```python
from build123d import *

# Parameters (mm, degrees)
BOSS_EXTRU_1_DEPTH      = 4
ENL_V_MAT_EXTRU_1_REACH = 44.274


with BuildPart() as part:
    # Esquisse1 → Boss.-Extru.1 (new body)
    with BuildSketch(Plane.XY):
        with BuildLine():
            Line((0, 0), (7, 0))
            Line((7, 0), (7, 4))
            Line((7, 4), (8.5, 4))
            add(Edge.make_bspline(
                [(8.5, 4), (8.5, 18.018365096), (18.5, 19.781634904), (18.5, 33.8)],
                knots=[0, 0, 0, 0, 1, 1, 1, 1], degree=3))
            Line((18.5, 33.8), (17, 33.8))
            Line((17, 33.8), (17, 37.8))
            Line((17, 37.8), (10, 37.8))
            Line((10, 37.8), (10, 33.8))
            Line((10, 33.8), (8.5, 33.8))
            add(Edge.make_bspline(
                [(-1.5, 4), (-1.5, 18.018365096), (8.5, 19.781634904), (8.5, 33.8)],
                knots=[0, 0, 0, 0, 1, 1, 1, 1], degree=3))
            Line((-1.5, 4), (0, 4))
            Line((0, 4), (0, 0))
        make_face()
    extrude(amount=BOSS_EXTRU_1_DEPTH)

    # Esquisse2 → Enlèv. mat.-Extru.1 (cut, up to next)
    with BuildSketch(Plane.XY.offset(4), mode=Mode.PRIVATE) as enl_v_mat_extru_1_sk1:
        with BuildLine():
            Line((11.098076211, 32.3), (15.901923789, 32.3))
            add(Edge.make_bspline(
                [(5.901923789, 5.5), (5.901923789, 16.568461709), (15.901923789, 21.231538291), (15.901923789, 32.3)],
                knots=[0, 0, 0, 0, 1, 1, 1, 1], degree=3))
            Line((5.901923789, 5.5), (1.098076211, 5.5))
            add(Edge.make_bspline(
                [(1.098076211, 5.5), (1.098076211, 16.568461709), (11.098076211, 21.231538291), (11.098076211, 32.3)],
                knots=[0, 0, 0, 0, 1, 1, 1, 1], degree=3))
        make_face()
    enl_v_mat_extru_1_tool1 = extrude(enl_v_mat_extru_1_sk1.sketch, amount=-ENL_V_MAT_EXTRU_1_REACH, mode=Mode.PRIVATE) & part.part
    add(enl_v_mat_extru_1_tool1.solids().sort_by_distance((8.5, 18.9, 4))[0], mode=Mode.SUBTRACT)


solid = part.part
```
Verification items for the finished model (mm, model axes). A direction names the side the tool comes from. Round coordinates to 2 decimals unless told otherwise and drop trailing zeros. Loops run counter-clockwise (first coordinate to the right, second up) from the corner with the lowest first, then second, coordinate; pieces in that order, holes last. Notation, with made-up numbers: (0.5, -5.75) -> (19.5, -5.75) arc R11 ccw to (19.5, 0.25) -> close; hole circle Ø11 at (15, 76). An arc over 180 degrees is marked (long way). Answer as a JSON object with one key per item and string values.
Q1. Draft check along X on faces 1 (the flat face through (13, 32.3, 2)), 2 (the flat face through (7, 2, 2)), 3 (the flat face through (18, 33.8, 2)). Enter one of: pulls with the +X half, pulls with the -X half, needs draft (parallel to the pull), parting line crosses it, or undercut.
Data:
{"face 1": "undercut", "face 2": "pulls with the +X half", "face 3": "needs draft"}
Q2. Scan lines: line 1 (X direction, y = 34.5, z = 3.8); line 2 (Y direction, x = 4.5, z = 0.9); line 3 (Y direction, x = 13.5, z = 3.3). Record each from-to range of solid material in increasing order. Write a range as from..to.
Data:
{"line 1": "x = 10..17", "line 2": "y = 0..5.5, 16.33..20.5", "line 3": "y = 18.9..23.25, 32.3..37.8"}
Q3. Go/stop test with flat-tipped pins: P1, Ø5, axis at x = 4.5, y = 20.5, coming from the -Z side; P2, Ø1.2, axis at x = 13.5, z = 2.5, coming from the -Y side; P3, Ø1.6, axis at x = 18, z = 2, coming from the +Y side; P4, Ø1.2, axis at x = 8, z = 2, coming from the -Y side. Record where each tip stops, or that it passes through.
Data:
{"P1": "stops at z = 0", "P2": "stops at y = 17.95", "P3": "stops at y = 33.8", "P4": "stops at y = 4"}
Q4. Access from +Z, -Z, +X, -X, +Y, -Y to the whole of each face (thin tool, end or side, straight path). Record for faces 4 (the flat face through (10, 36, 2)), 5 (the flat face through (0, 2, 2)), 6 (the flat face through (8, 4, 2)), 7 (the flat face through (17, 36, 2)), 8 (the flat face through (4, 5.5, 2)).
Data:
{"face 4": "+Z, -Z, -X, +Y", "face 5": "+Z, -Z, -X, -Y", "face 6": "+Z, -Z, +X, -Y", "face 7": "+Z, -Z, +X, +Y", "face 8": "+Z, -Z"}
Q5. Section check A-A (y = 35). Record the boundary of the cut face in (x, z).
Data:
{"outline": "(10, 0) -> (17, 0) -> (17, 4) -> (10, 4) -> close"}
